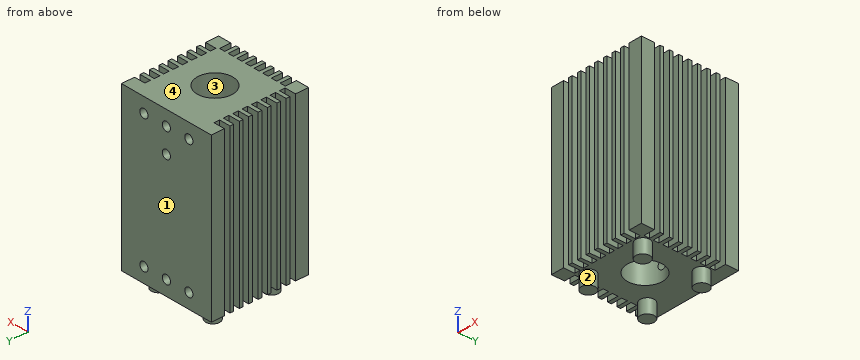
```python
from build123d import *

# Parameters (mm, degrees)
SKETCH1_W           = 33
SKETCH1_H           = 33
SKETCH1_R           = 6
BOSS_EXTRUDE1_DEPTH = 55
SKETCH2_R           = 1.5
CUT_EXTRUDE1_DEPTH  = 12.7
SKETCH5_W           = 3.81
SKETCH5_H           = 1.905
SKETCH5_W_2         = 1.905
SKETCH5_H_2         = 3.81
CUT_EXTRUDE2_DEPTH  = 56.0000001
SKETCH3_R           = 2.38125
BOSS_EXTRUDE2_DEPTH = 4.7625


with BuildPart() as part:
    # Sketch1 → Boss-Extrude1 (new body)
    with BuildSketch(Plane.XY):
        with Locations((16.5, 16.5)):
            Rectangle(SKETCH1_W, SKETCH1_H)
        with Locations((16.5, 16.5)):
            Circle(SKETCH1_R, mode=Mode.SUBTRACT)
    extrude(amount=-BOSS_EXTRUDE1_DEPTH)

    # Sketch2 → Cut-Extrude1 (cut)
    with BuildSketch(Plane(origin=(0, 33, 0), x_dir=(1, 0, 0), z_dir=(0, 1, 0))):
        with Locations((8.25, 5)):
            Circle(SKETCH2_R)
        with Locations((16.5, 5)):
            Circle(SKETCH2_R)
        with Locations((24.75, 5)):
            Circle(SKETCH2_R)
        with Locations((8.25, 50)):
            Circle(SKETCH2_R)
        with Locations((16.5, 50)):
            Circle(SKETCH2_R)
        with Locations((24.75, 50)):
            Circle(SKETCH2_R)
        with Locations((16.5, 13.25)):
            Circle(SKETCH2_R)
    extrude(amount=-CUT_EXTRUDE1_DEPTH, mode=Mode.SUBTRACT)

    # Sketch5 → Cut-Extrude2 (cut, through all)
    with BuildSketch(Plane.XY):
        with Locations((1.905, 27.6125)):
            Rectangle(SKETCH5_W, SKETCH5_H)
        with Locations((1.905, 24.4375)):
            Rectangle(SKETCH5_W, SKETCH5_H)
        with Locations((1.905, 21.2625)):
            Rectangle(SKETCH5_W, SKETCH5_H)
        with Locations((1.905, 18.0875)):
            Rectangle(SKETCH5_W, SKETCH5_H)
        with Locations((1.905, 14.9125)):
            Rectangle(SKETCH5_W, SKETCH5_H)
        with Locations((1.905, 11.7375)):
            Rectangle(SKETCH5_W, SKETCH5_H)
        with Locations((1.905, 8.5625)):
            Rectangle(SKETCH5_W, SKETCH5_H)
        with Locations((1.905, 5.3875)):
            Rectangle(SKETCH5_W, SKETCH5_H)
        with Locations((5.3875, 1.905)):
            Rectangle(SKETCH5_W_2, SKETCH5_H_2)
        with Locations((8.5625, 1.905)):
            Rectangle(SKETCH5_W_2, SKETCH5_H_2)
        with Locations((11.7375, 1.905)):
            Rectangle(SKETCH5_W_2, SKETCH5_H_2)
        with Locations((14.9125, 1.905)):
            Rectangle(SKETCH5_W_2, SKETCH5_H_2)
        with Locations((18.0875, 1.905)):
            Rectangle(SKETCH5_W_2, SKETCH5_H_2)
        with Locations((21.2625, 1.905)):
            Rectangle(SKETCH5_W_2, SKETCH5_H_2)
        with Locations((24.4375, 1.905)):
            Rectangle(SKETCH5_W_2, SKETCH5_H_2)
        with Locations((27.6125, 1.905)):
            Rectangle(SKETCH5_W_2, SKETCH5_H_2)
        with Locations((31.095, 5.3875)):
            Rectangle(SKETCH5_W, SKETCH5_H)
        with Locations((31.095, 8.5625)):
            Rectangle(SKETCH5_W, SKETCH5_H)
        with Locations((31.095, 11.7375)):
            Rectangle(SKETCH5_W, SKETCH5_H)
        with Locations((31.095, 14.9125)):
            Rectangle(SKETCH5_W, SKETCH5_H)
        with Locations((31.095, 18.0875)):
            Rectangle(SKETCH5_W, SKETCH5_H)
        with Locations((31.095, 21.2625)):
            Rectangle(SKETCH5_W, SKETCH5_H)
        with Locations((31.095, 24.4375)):
            Rectangle(SKETCH5_W, SKETCH5_H)
        with Locations((31.095, 27.6125)):
            Rectangle(SKETCH5_W, SKETCH5_H)
    extrude(amount=-CUT_EXTRUDE2_DEPTH, mode=Mode.SUBTRACT)

    # Sketch3 → Boss-Extrude2 (add)
    with BuildSketch(Plane.XY.offset(-55)):
        with Locations((6.5, 26.5)):
            Circle(SKETCH3_R)
        with Locations((26.5, 26.5)):
            Circle(SKETCH3_R)
        with Locations((26.5, 6.5)):
            Circle(SKETCH3_R)
        with Locations((6.5, 6.5)):
            Circle(SKETCH3_R)
    extrude(amount=-BOSS_EXTRUDE2_DEPTH)


solid = part.part
```
Input: part model. Units: mm. Frame: model coordinates. Face numbers are marked on the shaded views. A direction names the side the tool comes from. Coordinates: 2 decimals unless noted, no trailing zeros. Loops run counter-clockwise (first coordinate to the right, second up) from the corner with the lowest first, then second, coordinate; pieces in that order, holes last. Notation, with made-up numbers: M 53.5,15 L 88.5,15 A18 cw 88.5,40 Z; hole C -13.5,3 d11. An arc over 180 degrees is marked long. Use a Markdown table: item, result. Add a question column.
1) Line query: L1, parallel to X at y = 27, z = -50; L2, parallel to Z at x = 8.25, y = 27.5; L3, parallel to X at y = 29, z = -50. Output: solid intervals per line, ascending. Write a range as from..to.
2) Section A-A, the plane y = 16.5. Return the cut outline in (x, z), plus the area to 4 significant figures.
3) Pin query (flat end, axial travel): P1, Ø1.8, axis at x = 16.5, z = -13.25, coming from the +Y side; P2, Ø1.5, axis at y = 24.5, z = -26, coming from the +X side; P3, Ø0.6, axis at x = 15, z = -23, coming from the -Y side. Return the tip coordinate at first contact, or that it passes through.
4) Section C-C, the plane x = 12. Return the cut outline in (y, z).
5) Set-up query: the marked faces 1 and 2. Return all of +Z, -Z, +X, -X, +Y, -Y with unobstructed straight access to the full face (end or side cutting, diameter ignored); none if empty.
6) Section D-D, the plane y = 3. Give the number of separate pieces and of enclosed holes in the cut face, plus the area to 3 significant figures.
7) Section B-B, the plane x = 24.75. Return the cut outline in (y, z).
8) Draft query along X for the marked faces 3 and 4. Return one class per face: +X half, -X half, draft (parallel to the pull), parting line (faces both ways), or undercut.
Answer below:
| question | item | result |
|---|---|---|
| 1 | L1 | 3.81..6.75, 9.75..15, 18..23.25, 26.25..29.19 |
| 1 | L2 | -59.76..-51.5, -48.5..-6.5, -3.5..0 |
| 1 | L3 | 0..6.75, 9.75..15, 18..23.25, 26.25..33 |
| 2 | outline | M 0,-55 L 10.5,-55 L 10.5,0 L 0,0 Z; M 22.5,-55 L 33,-55 L 33,0 L 22.5,0 Z |
| 2 | area | 1,155 mm2 |
| 3 | P1 | y = 10.57 |
| 3 | P2 | x = 29.19 |
| 3 | P3 | y = 3.81 |
| 4 | outline | M 3.81,-55 L 12.53,-55 L 12.53,0 L 3.81,0 Z; M 20.47,-55 L 33,-55 L 33,0 L 20.47,0 Z |
| 5 | face 1 | +Z, -Z, +X, -X, +Y |
| 5 | face 2 | -Z |
| 6 | separate pieces | 9 |
| 6 | enclosed holes | 0 |
| 6 | area | 977 mm2 |
| 7 | outline | M 3.81,-55 L 4.89,-55 L 4.89,-59.76 L 8.11,-59.76 L 8.11,-55 L 24.89,-55 L 24.89,-59.76 L 28.11,-59.76 L 28.11,-55 L 33,-55 L 33,-51.5 L 20.3,-51.5 L 20.3,-48.5 L 33,-48.5 L 33,-6.5 L 20.3,-6.5 L 20.3,-3.5 L 33,-3.5 L 33,0 L 3.81,0 Z |
| 8 | face 3 | undercut |
| 8 | face 4 | draft |
